Autodesk Inventor part; units mm, degrees
ref_plane "YZ Plane" through (0, 0, 0) normal (1, 0, 0) x (0, 1, 0)
ref_plane "XZ Plane" through (0, 0, 0) normal (0, 1, 0) x (-1, 0, 0)
ref_plane "XY Plane" through (0, 0, 0) normal (0, 0, 1) x (1, 0, 0)
sketch "Sketch1" plane through (0, 0, 0) normal (0, 1, 0) x (-1, 0, 0)
  line L0 (0, 0) -> (124, 0)
  line L1 (124, 0) -> (124, -26)
  line L2 (124, -26) -> (0, -26)
  line L3 (0, -26) -> (0, 0)
  circle A0 centre (10.0002, -12.5957) radius 3
  circle A1 centre (114, -12.5957) radius 3
  line L4 (0, 0) -> (124.0002, 0)
  line L5 (124.0002, 0) -> (124.0002, -2.5957)
  line L6 (124.0002, -2.5957) -> (117, -2.5957)
  line L7 (117, -2.5957) -> (117, -5.5957)
  line L8 (117, -5.5957) -> (124.0002, -5.5957)
  line L9 (124.0002, -5.5957) -> (124.0002, -19.5957)
  line L10 (124.0002, -19.5957) -> (117, -19.5957)
  line L11 (117, -19.5957) -> (117, -22.5957)
  line L12 (117, -22.5957) -> (124.0002, -22.5957)
  line L13 (124.0002, -22.5957) -> (124.0002, -26)
  line L14 (124.0002, -26) -> (0, -26)
  line L15 (0, -26) -> (0, -22.5957)
  line L16 (0, -22.5957) -> (7, -22.5957)
  line L17 (7, -22.5957) -> (7, -19.5957)
  line L18 (7, -19.5957) -> (0, -19.5957)
  line L19 (0, -19.5957) -> (0, -5.5957)
  line L20 (0, -5.5957) -> (7, -5.5957)
  line L21 (7, -5.5957) -> (7, -2.5957)
  line L22 (7, -2.5957) -> (0, -2.5957)
  line L23 (0, -2.5957) -> (0, 0)
  line L24 (31.0002, -9.0957) -> (28.0002, -9.0957)
  line L25 (28.0002, -9.0957) -> (28.0002, -16.0957)
  line L26 (28.0002, -16.0957) -> (31.0002, -16.0957)
  line L27 (31.0002, -16.0957) -> (31.0002, -9.0957)
  line L28 (31.0002, -5.5957) -> (22, -5.5957)
  line L29 (22, -5.5957) -> (22, -2.5957)
  line L30 (22, -2.5957) -> (54.5, -2.5957)
  line L31 (54.5, -2.5957) -> (54.5, -5.5957)
  line L32 (54.5, -5.5957) -> (31.0002, -5.5957)
  line L33 (28.0002, -19.5957) -> (54.5, -19.5957)
  line L34 (54.5, -19.5957) -> (54.5, -22.5957)
  line L35 (54.5, -22.5957) -> (22, -22.5957)
  line L36 (22, -22.5957) -> (22, -19.5957)
  line L37 (22, -19.5957) -> (28.0002, -19.5957)
  line L38 (69.5, -5.5957) -> (69.5, -2.5957)
  line L39 (69.5, -2.5957) -> (102, -2.5957)
  line L40 (102, -2.5957) -> (102, -5.5957)
  line L41 (102, -5.5957) -> (69.5, -5.5957)
  line L42 (93, -9.0957) -> (96, -9.0957)
  line L43 (96, -9.0957) -> (96, -16.0957)
  line L44 (96, -16.0957) -> (93, -16.0957)
  line L45 (93, -16.0957) -> (93, -9.0957)
  line L46 (96, -19.5957) -> (69.5, -19.5957)
  line L47 (69.5, -19.5957) -> (69.5, -22.5957)
  line L48 (69.5, -22.5957) -> (102, -22.5957)
  line L49 (102, -22.5957) -> (102, -19.5957)
  line L50 (102, -19.5957) -> (96, -19.5957)
  dimension "d0" = 124
  dimension "d1" = 26
  dimension "d4" = 124.0002
  dimension "d5" = 26
extrude "Extrusion1" add sketch "Sketch1" along normal blind 89 contours L0 L1 L6 L7 L8 L10 L11 L12 L2 L3 L16 L17 L18 L20 L21 L22 | L22 L21 L20 L3 | L1 L8 L7 L6 | L18 L17 L16 L3 | L1 L12 L11 L10 | A0 | A1 | L27 L26 L25 L24 | L28 L29 L30 L31 L32 | L33 L34 L35 L36 L37 | L38 L39 L40 L41 | L42 L43 L44 L45 | L50 L49 L48 L47 L46
sketch "Sketch2" plane through (0, 89, 0) normal (0, 1, 0) x (1, 0, 0)
  line L0 (0, 0) -> (-124, 0)
  line L1 (-124, 0) -> (-124, 26)
  line L2 (-124, 26) -> (0, 26)
  line L3 (0, 26) -> (0, 0)
  line L4 (-28.0002, 16.0957) -> (-31.0002, 16.0957)
  line L5 (-31.0002, 16.0957) -> (-31.0002, 9.0957)
  line L6 (-31.0002, 9.0957) -> (-28.0002, 9.0957)
  line L7 (-31.0002, 5.5957) -> (-22, 5.5957)
  circle A0 centre (-10.0002, 12.5957) radius 3
  line L8 (-54.5, 2.5957) -> (-54.5, 5.5957)
  line L9 (-22, 2.5957) -> (-54.5, 2.5957)
  line L10 (-69.5, 5.5957) -> (-69.5, 2.5957)
  circle A1 centre (-114, 12.5957) radius 3
  line L11 (0, 0) -> (-124.0002, 0)
  line L12 (-124.0002, 26) -> (0, 26)
  line L13 (-117, 5.5957) -> (-124.0002, 5.5957)
  line L14 (-117, 19.5957) -> (-117, 22.5957)
  line L15 (-124.0002, 5.5957) -> (-124.0002, 19.5957)
  line L16 (-124.0002, 19.5957) -> (-117, 19.5957)
  line L17 (-117, 2.5957) -> (-117, 5.5957)
  line L18 (-124.0002, 2.5957) -> (-117, 2.5957)
  line L19 (-124.0002, 0) -> (-124.0002, 2.5957)
  line L20 (-124.0002, 22.5957) -> (-124.0002, 26)
  line L21 (-117, 22.5957) -> (-124.0002, 22.5957)
  line L22 (-102, 19.5957) -> (-96, 19.5957)
  line L23 (-102, 22.5957) -> (-102, 19.5957)
  line L24 (-96, 16.0957) -> (-93, 16.0957)
  line L25 (-93, 16.0957) -> (-93, 9.0957)
  line L26 (-93, 9.0957) -> (-96, 9.0957)
  line L27 (-96, 9.0957) -> (-96, 16.0957)
  line L28 (-96, 19.5957) -> (-69.5, 19.5957)
  line L29 (-69.5, 2.5957) -> (-102, 2.5957)
  line L30 (-102, 2.5957) -> (-102, 5.5957)
  line L31 (-102, 5.5957) -> (-69.5, 5.5957)
  line L32 (-69.5, 22.5957) -> (-102, 22.5957)
  line L33 (-69.5, 19.5957) -> (-69.5, 22.5957)
  line L34 (-54.5, 5.5957) -> (-31.0002, 5.5957)
  line L35 (-28.0002, 9.0957) -> (-28.0002, 16.0957)
  line L36 (-54.5, 22.5957) -> (-22, 22.5957)
  line L37 (-28.0002, 19.5957) -> (-54.5, 19.5957)
  line L38 (-54.5, 19.5957) -> (-54.5, 22.5957)
  line L39 (-22, 19.5957) -> (-28.0002, 19.5957)
  line L40 (-22, 22.5957) -> (-22, 19.5957)
  line L41 (-22, 5.5957) -> (-22, 2.5957)
  line L42 (0, 26) -> (0, 22.5957)
  line L43 (0, 22.5957) -> (-7, 22.5957)
  line L44 (-7, 22.5957) -> (-7, 19.5957)
  line L45 (-7, 19.5957) -> (0, 19.5957)
  line L46 (0, 19.5957) -> (0, 5.5957)
  line L47 (0, 5.5957) -> (-7, 5.5957)
  line L48 (-7, 2.5957) -> (0, 2.5957)
  line L49 (0, 2.5957) -> (0, 0)
  line L50 (-7, 5.5957) -> (-7, 2.5957)
  dimension "d6" = 124
  dimension "d7" = 26
  dimension "d8" = 124.0002
  dimension "d9" = 26
extrude "Extrusion2" cut sketch "Sketch2" against normal blind 10 contours A0 | A1
thread "Thread1"
thread "Thread2"
properties part number "base_soportes"
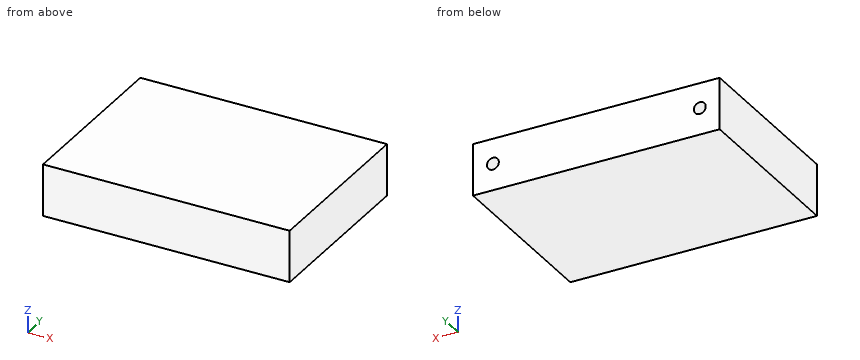
Design review of the part built by this model. Coordinates are the model's own, in mm. Round coordinates to 2 decimals unless told otherwise and drop trailing zeros. Loops run counter-clockwise (first coordinate to the right, second up) from the corner with the lowest first, then second, coordinate; pieces in that order, holes last. Notation, with made-up numbers: (44, 5.5) - (94, 5.5) arc R10 cw to (94, 14.5) - close; hole circle Ø1 at (21, 30.25). An arc over 180 degrees is marked (long way). One line per item, written item: value. Start each with the question number.
1) Consider section A-A on x = -114. Give the boundary of the cut face in (y, z), then the cut area to 3 significant figures.
2) Insertion check: pin 1 Ø1.5 at (x, z) = (-62, -4) entering from -Y; pin 2 Ø5.5 at (x, z) = (-10, -12.6) entering from +Y. Each pin has a flat end and moves straight along its axis. Give the tip position at first contact, or say it passes through.
3) To check wall thickness, follow L1, parallel to Z at x = -114, y = 83; L2, parallel to X at y = 81, z = -13.5; L3, parallel to X at y = 85.5, z = -13.75. State the ranges of each line that lie inside material, in increasing order. Write a range as from..to.
Reported:
1. outline: (0, -26) - (89, -26) - (89, -15.6) - (79, -15.6) - (79, -9.6) - (89, -9.6) - (89, 0) - (0, 0) - close
1. area: 2,250 mm^2
2. pin 1: stops at y = 0
2. pin 2: stops at y = 79
3. L1: z = -26..-15.6, -9.6..0
3. L2: x = -124..-116.86, -111.14..-12.86, -7.14..0
3. L3: x = -124..-116.77, -111.23..-12.77, -7.23..0
